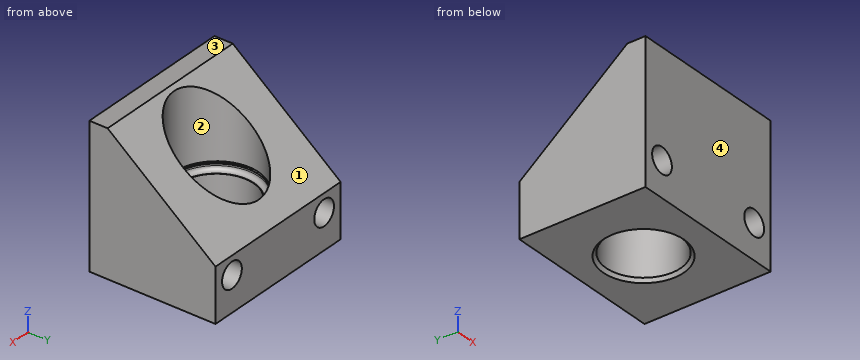
```python
from build123d import *

# Parameters (mm, degrees)
SKETCH1_W          = 56.9976
SKETCH1_H          = 44.9834
SKETCH1_R          = 13.259
EXTRUDE1_DEPTH     = 49.9872
CUT_EXTRUDE1_DEPTH = 57.9976
SKETCH3_R          = 15.113
CUT_EXTRUDE2_DEPTH = 30.988
FILLET1_R          = 1.524
HOLE1_D            = 8.9916
HOLE1_DEPTH        = 44.9834


with BuildPart() as part:
    # Sketch1 → Extrude1 (new body)
    with BuildSketch(Plane.XY):
        with Locations((28.4988, 22.4917)):
            Rectangle(SKETCH1_W, SKETCH1_H)
        with Locations((28.4988, 23.0124)):
            Circle(SKETCH1_R, mode=Mode.SUBTRACT)
    extrude(amount=-EXTRUDE1_DEPTH)

    # Sketch2 → Cut-Extrude1 (cut, through all)
    with BuildSketch(Plane(origin=(56.9976, 0, 0), x_dir=(0, 0, -1), z_dir=(1, 0, 0))):
        Polygon((0, 44.9834), (30.988, 44.9834), (0, 6.5024), align=None)
    extrude(amount=-CUT_EXTRUDE1_DEPTH, mode=Mode.SUBTRACT)

    # Sketch3 → Cut-Extrude2 (cut)
    with BuildSketch(Plane(origin=(0, 0, 0), x_dir=(-1, 0, 0), z_dir=(0, 0, -1))):
        with Locations(Location((-28.4988, 23.0124, 0), (0, 0, 180))):  # turned: the seam where the file's is
            Circle(SKETCH3_R)
    extrude(amount=CUT_EXTRUDE2_DEPTH, mode=Mode.SUBTRACT)

    # Fillet1
    fillet1_edges = [part.edges().sort_by_distance(p)[0] for p in [
        (13.3858, 23.0124, -30.988),
    ]]
    fillet(fillet1_edges, radius=FILLET1_R)

    # Hole1
    with Locations(Plane(origin=(0, 44.9834, 0), x_dir=(-1, 0, 0), z_dir=(0, 1, 0))):
        with Locations((-7.5184, -37.4904), (-49.5046, -37.4904)):
            Hole(HOLE1_D / 2, depth=HOLE1_DEPTH)

    # Sketch6 → Cut-Revolve1 (revolve, cut)
    with BuildSketch(Plane(origin=(0, 23.0124, 0), x_dir=(-1, 0, 0), z_dir=(0, 1, 0)), mode=Mode.PRIVATE) as cut_revolve1_sk:
        Polygon((-13.3858, -28.0162), (-13.3858, -28.7782), (-13.0048, -28.3972), align=None)
        Polygon((-15.2398, -48.8952), (-15.2398, -49.9872), (-14.1478, -49.9872), align=None)
    revolve(cut_revolve1_sk.sketch.rotate(Axis((28.4988, 23.0124, 17.508123997), (0, 0, -1)), 180), axis=Axis((28.4988, 23.0124, 17.508123997), (0, 0, -1)), mode=Mode.SUBTRACT)  # turned: the seam where the file's is


solid = part.part
```
Input: part model. Units: mm. Frame: model coordinates. Face numbers are marked on the shaded views. Coordinates: 2 decimals unless noted, no trailing zeros. Write each loop counter-clockwise with the first axis right and the second up, starting at its lowest first coordinate (ties: lowest second). Pieces come first, ordered by that corner, then holes. Notation, with made-up numbers: (24.5, 57) -> (32.5, 57) arc R19 ccw to (32.5, 86) -> close; hole circle Ø7 at (-5, 28). An arc over 180 degrees is marked (long way). Answer as a JSON object with one key per item and string values.
1. First-contact query: P1, Ø12, axis at y = 26.5, z = -6, coming from the -X side; P2, Ø1, axis at x = 41, z = -20, coming from the +Y side; P3, Ø1, axis at x = 37, z = -8, coming from the +Y side. Flat tips, straight axial feed; report the tip coordinate or a pass-through.
Result set:
{"P1": "passes through", "P2": "stops at y = 31.96", "P3": "stops at y = 10.87"}
2. Mould query, pull axis Y, two halves, no side actions, for the marked faces 1, 2, 3 and 4. Classes: released by +Y, released by -Y, zero draft, split by the parting line, or undercut.
Result set:
{"face 1": "released by +Y", "face 2": "undercut", "face 3": "zero draft", "face 4": "released by -Y"}
3. Material intervals for line 1 (X direction, y = 17, z = -38.5); line 2 (Y direction, x = 41, z = -24); line 3 (Z direction, x = 7, y = 12.5), sorted ascending. Write a range as from..to.
Result set:
{"line 1": "x = 0..3.14, 11.9..16.68, 40.32..45.12, 53.89..57", "line 2": "y = 0..14.52, 31.5..36.31", "line 3": "z = -49.99..-41.96, -33.02..-4.83"}
4. Section B-B on x = 8.5. Return the cut outline in (y, z), then the cut area to 3 significant figures.
Result set:
{"outline": "(0, -49.99) -> (44.98, -49.99) -> (44.98, -41.88) -> (0, -41.88) -> close; (0, -33.1) -> (44.98, -33.1) -> (44.98, -30.99) -> (6.5, 0) -> (0, 0) -> close", "area": "1,260 mm2"}
5. Section C-C on y = 41.5. Return the cut outline in (x, z), then the cut area to 3 significant figures.
Result set:
{"outline": "(0, -49.99) -> (57, -49.99) -> (57, -28.18) -> (0, -28.18) -> close; hole circle Ø8.99 at (7.52, -37.49); hole circle Ø8.99 at (49.5, -37.49)", "area": "1,120 mm2"}
6. Section D-D on y = 31. Count the separate pieces of the cut face and the enclosed holes in it, then the cut area to 3 significant figures.
Result set:
{"separate pieces": "2", "enclosed holes": "2", "area": "906 mm2"}
7. Section A-A on z = -36. Return the cut outline in (x, y).
Result set:
{"outline": "(0, 0) -> (3.28, 0) -> (3.28, 44.98) -> (0, 44.98) -> close; (11.76, 0) -> (45.26, 0) -> (45.26, 44.98) -> (11.76, 44.98) -> close; (53.75, 0) -> (57, 0) -> (57, 44.98) -> (53.75, 44.98) -> close; hole circle Ø26.52 at (28.5, 23.01)"}
